Model file for the job. Use its own axes, mm. A direction names the side the tool comes from. Round coordinates to 2 decimals unless told otherwise and drop trailing zeros. Order: outer loops, then holes, each group sorted by start corner. A loop starts at its lowest first (then second) coordinate and runs counter-clockwise, first axis right, second up. Notation, with made-up numbers: (71.25, 57) - (84.25, 57) arc R18 ccw to (84.25, 79) - close; hole circle Ø8 at (65.5, -2). An arc over 180 degrees is marked (long way). Put each result on its own line as item: value. Start each with the question number.
Item 1: Probe probe 1 along Y at (x, z) = (328, 12.5); probe 2 along X at (y, z) = (-15, 42.5); probe 3 along X at (y, z) = (-23, 35.5). List the from-to ranges inside material, lowest first.
Item 2: Saw through at A-A on y = -15. List the corners of the cut face in (x, z), plus the area to 3 significant figures.
Item 3: Which spindle directions (+Z, -Z, +X, -X, +Y, -Y) get a long thin tool onto all of the face, cutting with end or side? Do faces 1 (the face through (865, -15, 39)), 2 (the face through (47, -33, 39)). Say none if no direction does.
Item 4: Pin check, flat tip, straight feed: pin 1 Ø4 at (y, z) = (-29, 32.5) entering from +X. Stop position of the tip, or through.
Item 5: Mould opens along X. For faces 3 (the face through (533, -33, 39)), 4 (the face through (-15, -15, 39)), 5 (the face through (868, -15, 39)) say: pulls with the +X half, pulls with the -X half, needs draft (parallel to the pull), parting line crosses it, or undercut.
```python
from build123d import *

# Parameters (mm, degrees)
EXTRUIR_L_MINA1_DEPTH        = 80
CROQUIS4_W                   = 1
CROQUIS4_H                   = 80
CORTAR_EXTRUIR_L_MINA1_DEPTH = 1
CROQUIS5_W                   = 1
CROQUIS5_H                   = 80
CORTAR_EXTRUIR_L_MINA2_DEPTH = 1


with BuildPart() as part:
    # Croquis1 → Extruir-Lámina1 (new body)
    with BuildSketch(Plane.XY):
        with BuildLine():
            Line((0, 3), (850, 3))
            ThreePointArc((850, 3), (868, -15), (850, -33))
            Line((850, -33), (0, -33))
            ThreePointArc((0, -33), (-18, -15), (0, 3))
        make_face()
        with BuildLine():
            Line((0, 0), (850, 0))
            ThreePointArc((850, 0), (865, -15), (850, -30))
            Line((850, -30), (0, -30))
            ThreePointArc((0, -30), (-15, -15), (0, 0))
        make_face(mode=Mode.SUBTRACT)
    extrude(amount=EXTRUIR_L_MINA1_DEPTH)

    # Croquis4 → Cortar-Extruir-Lámina1 (cut)
    with BuildSketch(Plane(origin=(0, 3, 0), x_dir=(1, 0, 0), z_dir=(0, 1, 0))):
        with Locations((424.5, -40)):
            Rectangle(CROQUIS4_W, CROQUIS4_H)
        with Locations((65.374468325, -40)):
            Rectangle(CROQUIS4_W, CROQUIS4_H)
        with Locations((145.374468325, -40)):
            Rectangle(CROQUIS4_W, CROQUIS4_H)
        with Locations((225.374468325, -40)):
            Rectangle(CROQUIS4_W, CROQUIS4_H)
        with Locations((305.374468325, -40)):
            Rectangle(CROQUIS4_W, CROQUIS4_H)
        with Locations((385.374468325, -40)):
            Rectangle(CROQUIS4_W, CROQUIS4_H)
        with Locations((465.374468325, -40)):
            Rectangle(CROQUIS4_W, CROQUIS4_H)
        with Locations((545.374468325, -40)):
            Rectangle(CROQUIS4_W, CROQUIS4_H)
        with Locations((625.374468325, -40)):
            Rectangle(CROQUIS4_W, CROQUIS4_H)
        with Locations((705.374468325, -40)):
            Rectangle(CROQUIS4_W, CROQUIS4_H)
        with Locations((785.374468325, -40)):
            Rectangle(CROQUIS4_W, CROQUIS4_H)
    extrude(amount=-CORTAR_EXTRUIR_L_MINA1_DEPTH, mode=Mode.SUBTRACT)

    # Croquis5 → Cortar-Extruir-Lámina2 (cut)
    with BuildSketch(Plane.XZ.offset(33)):
        with Locations((92.409174229, 40)):
            Rectangle(CROQUIS5_W, CROQUIS5_H)
        with Locations((172.409174229, 40)):
            Rectangle(CROQUIS5_W, CROQUIS5_H)
        with Locations((252.409174229, 40)):
            Rectangle(CROQUIS5_W, CROQUIS5_H)
        with Locations((332.409174229, 40)):
            Rectangle(CROQUIS5_W, CROQUIS5_H)
        with Locations((412.409174229, 40)):
            Rectangle(CROQUIS5_W, CROQUIS5_H)
        with Locations((492.409174229, 40)):
            Rectangle(CROQUIS5_W, CROQUIS5_H)
        with Locations((572.409174229, 40)):
            Rectangle(CROQUIS5_W, CROQUIS5_H)
        with Locations((652.409174229, 40)):
            Rectangle(CROQUIS5_W, CROQUIS5_H)
        with Locations((732.409174229, 40)):
            Rectangle(CROQUIS5_W, CROQUIS5_H)
        with Locations((812.409174229, 40)):
            Rectangle(CROQUIS5_W, CROQUIS5_H)
    extrude(amount=-CORTAR_EXTRUIR_L_MINA2_DEPTH, mode=Mode.SUBTRACT)


solid = part.part
```
Results found:
1. probe 1: y = -33 to -30, 0 to 3
1. probe 2: x = -18 to -15, 865 to 868
1. probe 3: x = -16.12 to -12.69, 862.69 to 866.12
2. outline: (-18, 0) - (-15, 0) - (-15, 80) - (-18, 80) - close; (865, 0) - (868, 0) - (868, 80) - (865, 80) - close
2. area: 480 mm²
3. face 1: +Z, -Z
3. face 2: +Z, -Z, +X, -X, -Y
4. pin 1: stops at x = 863.42
5. face 3: needs draft
5. face 4: undercut
5. face 5: pulls with the +X half
